Geometry check sheet. Reference: drawing and pictorial views, mm from the part's lowest x, y, z. Round coordinates to 2 decimals unless told otherwise and drop trailing zeros. Write each loop counter-clockwise with the first axis right and the second up, starting at its lowest first coordinate (ties: lowest second). Pieces come first, ordered by that corner, then holes. Notation, with made-up numbers: (-13.5, 17) -> (-7.5, 17) arc R11 cw to (-7.5, 37) -> close; hole circle Ø3 at (-32.5, 88.5). An arc over 180 degrees is marked (long way). Write item = value, one per line.
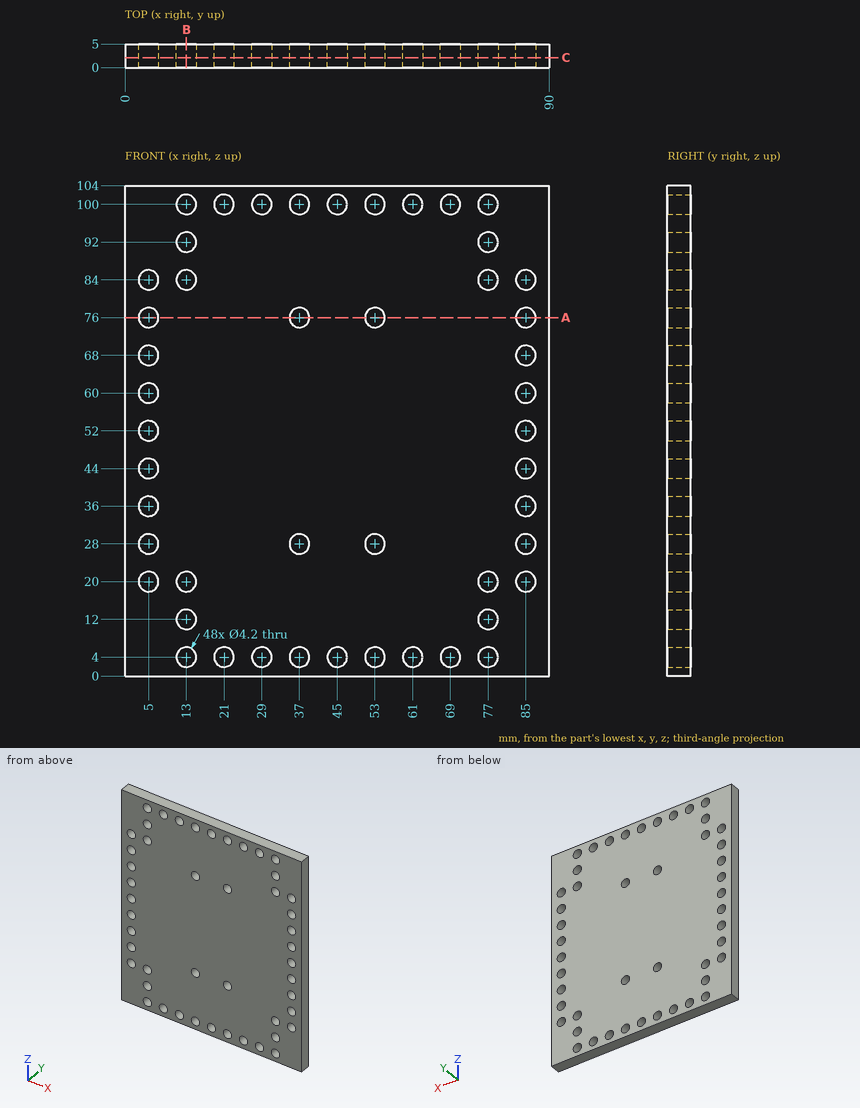
(1) Sectioned sample at C-C on y = 2.1. Count the separate pieces of the cut face and the enclosed holes in it, then the cut area to 4 significant figures.
Worked answers:
separate_pieces = 1
enclosed_holes = 48
area = 8,695 mm²
(2) Material ranges on L1, parallel to Z at x = 61, y = 2.05; L2, parallel to Z at x = 37, y = 2.25; L3, parallel to Z at x = 52.5, y = 0.9, recorded low to high. Write a range as [from, to].
Worked answers:
L1 = [0, 1.9], [6.1, 97.9], [102.1, 104]
L2 = [0, 1.9], [6.1, 25.9], [30.1, 73.9], [78.1, 97.9], [102.1, 104]
L3 = [0, 1.96], [6.04, 25.96], [30.04, 73.96], [78.04, 97.96], [102.04, 104]
(3) Sectioned sample at B-B on x = 13. Enter the section's corners in (y, z).
Worked answers:
outline = (0, 0) -> (5, 0) -> (5, 1.9) -> (0, 1.9) -> close; (0, 6.1) -> (5, 6.1) -> (5, 9.9) -> (0, 9.9) -> close; (0, 14.1) -> (5, 14.1) -> (5, 17.9) -> (0, 17.9) -> close; (0, 22.1) -> (5, 22.1) -> (5, 81.9) -> (0, 81.9) -> close; (0, 86.1) -> (5, 86.1) -> (5, 89.9) -> (0, 89.9) -> close; (0, 94.1) -> (5, 94.1) -> (5, 97.9) -> (0, 97.9) -> close; (0, 102.1) -> (5, 102.1) -> (5, 104) -> (0, 104) -> close
(4) Sectioned sample at A-A on z = 76. Enter the section's corners in (x, y).
Worked answers:
outline = (0, 0) -> (2.9, 0) -> (2.9, 5) -> (0, 5) -> close; (7.1, 0) -> (34.9, 0) -> (34.9, 5) -> (7.1, 5) -> close; (39.1, 0) -> (50.9, 0) -> (50.9, 5) -> (39.1, 5) -> close; (55.1, 0) -> (82.9, 0) -> (82.9, 5) -> (55.1, 5) -> close; (87.1, 0) -> (90, 0) -> (90, 5) -> (87.1, 5) -> close
